Input: part model. Units: mm. Frame: model coordinates. A direction names the side the tool comes from. Give positions to 0.01 mm unless a question says otherwise; leave off trailing zeros. Loops run counter-clockwise (first coordinate to the right, second up) from the corner with the lowest first, then second, coordinate; pieces in that order, holes last. Notation, with made-up numbers: (71.5, 40.5) - (89.5, 40.5) arc R5 ccw to (89.5, 44.5) - close; hole circle Ø11 at (-14.5, -27). An arc over 180 degrees is marked (long way). One line per item, written item: value.
from build123d import *

# Parameters (mm, degrees)
ESBO_O1_W             = 20
ESBO_O1_H             = 70
FLANGE_BASE1_DEPTH    = 20
ESBO_O3_R             = 4.775
CORTE_EXTRUS_O1_DEPTH = 5.75
ESBO_O4_R             = 2.65
CORTE_EXTRUS_O2_DEPTH = 40.090440008
ESBO_O5_R             = 4
ESBO_O5_R_2           = 3
CORTE_EXTRUS_O3_DEPTH = 46
CORTE_EXTRUS_O5_REACH = 43.533
ESBO_O6_R             = 1.65


# Sheet-metal steps are written as plain solids
with BuildPart() as part:
    # Esboço1 → Flange-base1 (new body)
    with BuildSketch(Plane(origin=(0, 0, 0), x_dir=(1, 0, 0), z_dir=(0, 1, 0))):
        Rectangle(ESBO_O1_W, ESBO_O1_H)
    extrude(amount=-FLANGE_BASE1_DEPTH)

    # Esboço3 → Corte-extrusão1 (cut)
    with BuildSketch(Plane(origin=(0, 0, 0), x_dir=(1, 0, 0), z_dir=(0, 1, 0))):
        with Locations(Location((0, 13, 0), (0, 0, 270))):
            Circle(ESBO_O3_R)
        with Locations(Location((0, -13, 0), (0, 0, 270))):
            Circle(ESBO_O3_R)
    extrude(amount=-CORTE_EXTRUS_O1_DEPTH, mode=Mode.SUBTRACT)

    # Esboço4 → Corte-extrusão2 (cut, through all)
    with BuildSketch(Plane(origin=(0, -5.75, 0), x_dir=(1, 0, 0), z_dir=(0, 1, 0))):
        with Locations(Location((0, 13, 0), (0, 0, 270))):
            Circle(ESBO_O4_R)
        with Locations(Location((0, -13, 0), (0, 0, 270))):
            Circle(ESBO_O4_R)
    extrude(amount=-CORTE_EXTRUS_O2_DEPTH, mode=Mode.SUBTRACT)

    # Esboço5 → Corte-extrusão3 (cut, through all)
    with BuildSketch(Plane(origin=(10, 0, 0), x_dir=(0, 0, -1), z_dir=(1, 0, 0))):
        with Locations((-26, -10)):
            Circle(ESBO_O5_R)
        with Locations((26, -10)):
            Circle(ESBO_O5_R)
        with Locations((0, -10)):
            Circle(ESBO_O5_R_2)
    extrude(amount=-CORTE_EXTRUS_O3_DEPTH, mode=Mode.SUBTRACT)

    # Esboço6 → Corte-extrusão5 (cut, up to next)
    with BuildSketch(Plane(origin=(0, 0, 0), x_dir=(1, 0, 0), z_dir=(0, 1, 0)), mode=Mode.PRIVATE) as corte_extrus_o5_sk1:
        with Locations(Location((0, -26, 0), (0, 0, 270))):
            Circle(ESBO_O6_R)
    corte_extrus_o5_tool1 = extrude(corte_extrus_o5_sk1.sketch, amount=-CORTE_EXTRUS_O5_REACH, mode=Mode.PRIVATE) & part.part
    # Esboço6 → Corte-extrusão5 (cut, up to next)
    with BuildSketch(Plane(origin=(0, 0, 0), x_dir=(1, 0, 0), z_dir=(0, 1, 0)), mode=Mode.PRIVATE) as corte_extrus_o5_sk2:
        with Locations(Location((0, 26, 0), (0, 0, 270))):
            Circle(ESBO_O6_R)
    corte_extrus_o5_tool2 = extrude(corte_extrus_o5_sk2.sketch, amount=-CORTE_EXTRUS_O5_REACH, mode=Mode.PRIVATE) & part.part
    # Esboço6 → Corte-extrusão5 (cut, up to next)
    with BuildSketch(Plane(origin=(0, 0, 0), x_dir=(1, 0, 0), z_dir=(0, 1, 0)), mode=Mode.PRIVATE) as corte_extrus_o5_sk3:
        with Locations(Location((0, 0, 0), (0, 0, 270))):
            Circle(ESBO_O6_R)
    corte_extrus_o5_tool3 = extrude(corte_extrus_o5_sk3.sketch, amount=-CORTE_EXTRUS_O5_REACH, mode=Mode.PRIVATE) & part.part
    add(corte_extrus_o5_tool1.solids().sort_by_distance((0, 0, 26))[0], mode=Mode.SUBTRACT)
    add(corte_extrus_o5_tool2.solids().sort_by_distance((0, 0, -26))[0], mode=Mode.SUBTRACT)
    add(corte_extrus_o5_tool3.solids().sort_by_distance((0, 0, 0))[0], mode=Mode.SUBTRACT)


solid = part.part
Item 1: Material intervals for L1, parallel to X at y = -4.5, z = -13 (3 decimals); L2, parallel to Z at x = 8, y = -9; L3, parallel to X at y = -9.5, z = -13, sorted ascending.
Verdict:
L1: x = -10 to -4.775, 4.775 to 10
L2: z = -35 to -29.87, -22.13 to -2.83, 2.83 to 22.13, 29.87 to 35
L3: x = -10 to -2.65, 2.65 to 10
Item 2: Section B-B, the plane y = -10. Output: boundary loops of the cut face in (x, z), and give its area (3 significant figures).
Verdict:
outline: (-10, -35) - (10, -35) - (10, -30) - (-10, -30) - close; (-10, -22) - (10, -22) - (10, -3) - (-10, -3) - close; (-10, 3) - (10, 3) - (10, 22) - (-10, 22) - close; (-10, 30) - (10, 30) - (10, 35) - (-10, 35) - close; hole circle Ø5.3 at (0, -13); hole circle Ø5.3 at (0, 13)
area: 916 mm^2
Item 3: Access query for faces 1 (the face through (0.07, -3.13, 24.35)), 2 (the face through (0, -10, -35)). Directions: +Z, -Z, +X, -X, +Y, -Y. A direction counts if a zero-diameter tool reaches every point of the face in a straight line with its end or side. Return the directions, or none.
Verdict:
face 1: +Y
face 2: -Z, +X, -X, +Y, -Y
Item 4: Pin query (flat end, axial travel): P1, Ø2.5, axis at x = 0, z = -26, coming from the +Y side; P2, Ø7.5, axis at x = 0, z = 13, coming from the +Y side; P3, Ø3, axis at x = 0, z = 13, coming from the +Y side; P4, Ø2.5, axis at x = 0, z = 0, coming from the +Y side. Return the tip coordinate at first contact, or that it passes through.
Verdict:
P1: stops at y = -13.8
P2: stops at y = -5.75
P3: passes through
P4: stops at y = -12.73
Item 5: Section C-C, the plane x = 0. Count the separate pieces of the cut face and the enclosed holes in it, and give its area (3 significant figures).
Verdict:
separate pieces: 3
enclosed holes: 0
area: 946 mm^2
Item 6: Draft query along Z for faces 3 (the face through (0.14, -13.905, -25.133)), 4 (the face through (0.796, -12.775, 15.528)), 5 (the face through (0, -10, 35)), 6 (the face through (0, -20, 0)). Return one class per face: pulls with the +Z half, pulls with the -Z half, needs draft (parallel to the pull), parting line crosses it, or undercut.
Verdict:
face 3: undercut
face 4: undercut
face 5: pulls with the +Z half
face 6: needs draft
Item 7: Section D-D, the plane z = -13. Output: boundary loops of the cut face in (x, y) (3 decimals), and give its area (3 significant figures).
Verdict:
outline: (-10, -20) - (-2.65, -20) - (-2.65, -5.75) - (-4.775, -5.75) - (-4.775, 0) - (-10, 0) - close; (2.65, -20) - (10, -20) - (10, 0) - (4.775, 0) - (4.775, -5.75) - (2.65, -5.75) - close
area: 270 mm^2
Item 8: Section A-A, the plane z = 0. Output: boundary loops of the cut face in (x, y).
Verdict:
outline: (-10, -20) - (10, -20) - (10, -13) - (-10, -13) - close; (-10, -7) - (-1.65, -7) - (-1.65, 0) - (-10, 0) - close; (1.65, -7) - (10, -7) - (10, 0) - (1.65, 0) - close
